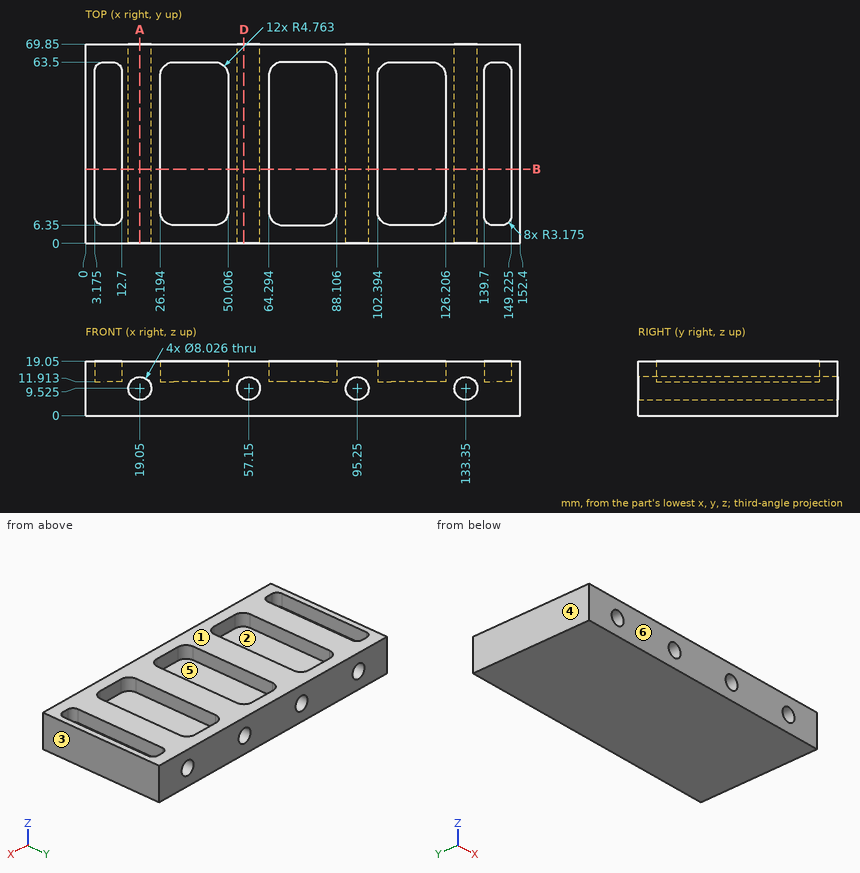
For this review, use the dimensioned drawing (mm, ordinates from the lowest corner) and the shaded views. A direction names the side the tool comes from. Give positions to 0.01 mm unless a question says otherwise; leave off trailing zeros. Write each loop counter-clockwise with the first axis right and the second up, starting at its lowest first coordinate (ties: lowest second). Pieces come first, ordered by that corner, then holes. Notation, with made-up numbers: M 34.25,22 L 55.25,22 A26 ccw 55.25,56 Z; hole C -15,73 d3. An arc over 180 degrees is marked long. Answer as a JSON object with one key per item and string values. Group by question number.
Item 1: Consider section A-A on x = 19.05. Write out the cut boundary in (y, z).
Item 2: Draft analysis for pull direction X (two halves, no side actions). For the marked faces 1, 2, 3 and 4, state which applies: +X half, -X half, draft (parallel to the pull), parting line (faces both ways), or undercut.
Item 3: Consider section B-B on y = 26. Count the separate pieces of the cut face and the enclosed holes in it.
Item 4: For probe 1 along X at (y, z) = (12, 17.25) (1 decimal); probe 2 along Z at (x, y) = (95, 40); probe 3 along Y at (x, z) = (70, 13.5), list the stretches that pass through material, from the lowest coordinate up. Write a range as [from, to].
Item 5: Tool access review of the marked faces 5 and 6: name each direction out of +Z, -Z, +X, -X, +Y, -Y from which nothing blocks a thin tool from reaching the whole face with its end or side.
Item 6: For pin 1 Ø7 at (x, y) = (108.5, 40.5) entering from +Z, flat-tipped, find the tip position at first contact; note if it passes through.
Item 7: Consider section D-D on x = 55.5. Write out the cut boundary in (y, z).
Check result:
{
 "1": {"outline": "M 0,0 L 69.85,0 L 69.85,5.51 L 0,5.51 Z; M 0,13.54 L 69.85,13.54 L 69.85,19.05 L 0,19.05 Z"},
 "2": {"face 1": "draft", "face 2": "undercut", "face 3": "+X half", "face 4": "-X half"},
 "3": {"separate pieces": "1", "enclosed holes": "4"},
 "4": {"probe 1": "x = [0, 3.2], [12.7, 26.2], [50, 64.3], [88.1, 102.4], [126.2, 139.7], [149.2, 152.4]", "probe 2": "z = [0, 5.52], [13.53, 19.05]", "probe 3": "y = [0, 6.35], [63.5, 69.85]"},
 "5": {"face 5": "+Z", "face 6": "+Z, -Z, +X, -X, -Y"},
 "6": {"pin 1": "stops at z = 11.91"},
 "7": {"outline": "M 0,0 L 69.85,0 L 69.85,5.87 L 0,5.87 Z; M 0,13.18 L 69.85,13.18 L 69.85,19.05 L 0,19.05 Z"}
}
